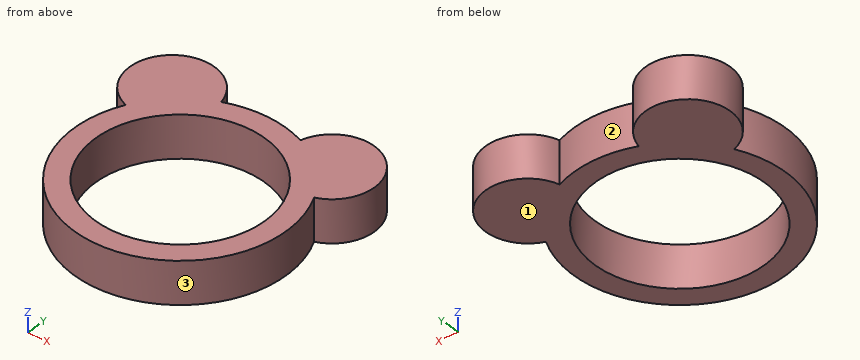
```python
from build123d import *

# Parameters (mm, degrees)
CYLINDER001_R     = 4
CYLINDER001_DEPTH = 5
CYLINDER003_R     = 2
CYLINDER003_DEPTH = 2
CYLINDER002_R     = 2
CYLINDER002_DEPTH = 2
CYLINDER_R        = 5
CYLINDER_DEPTH    = 2


with BuildPart() as interior:
    # Cylinder001 → Cylinder001 (new body)
    with BuildSketch(Plane.XY.offset(-1.53)):
        Circle(CYLINDER001_R)
    extrude(amount=CYLINDER001_DEPTH)


with BuildPart() as obj1:
    # Cylinder003 → Cylinder003 (new body)
    with BuildSketch(Plane(origin=(3.74, 4.15, 0), x_dir=(1, 0, 0), z_dir=(0, 0, 1))):
        Circle(CYLINDER003_R)
    extrude(amount=CYLINDER003_DEPTH)


with BuildPart() as cut001:
    # Cylinder002 → Cylinder002 (new body)
    with BuildSketch(Plane(origin=(-3.86, 4.15, 0), x_dir=(1, 0, 0), z_dir=(0, 0, 1))):
        Circle(CYLINDER002_R)
    extrude(amount=CYLINDER002_DEPTH)

    # Fusion: union obj1
    add(obj1.part)

    # Cut001: cut Interior
    add(interior.part, mode=Mode.SUBTRACT)


with BuildPart() as fusion001:
    # Cylinder → Cylinder (new body)
    with BuildSketch(Plane.XY):
        Circle(CYLINDER_R)
    extrude(amount=CYLINDER_DEPTH)

    # Cut: cut Interior
    add(interior.part, mode=Mode.SUBTRACT)

    # Fusion001: union Cut001
    add(cut001.part)


solid = fusion001.part
```
Can you work these out from the model? Positions are in its coordinate system, mm. Face numbers are marked on the shaded views. Give positions to 0.01 mm unless a question says otherwise; leave off trailing zeros. Order: outer loops, then holes, each group sorted by start corner. A loop starts at its lowest first (then second) coordinate and runs counter-clockwise, first axis right, second up. Notation, with made-up numbers: (85, 25.25) - (136, 25.25) arc R12 ccw to (136, 32.25) - close; hole circle Ø6 at (-3.5, 0). An arc over 180 degrees is marked (long way). Use a Markdown table: item, result. Add a question column.
Q1. If we section it at C-C on z = 0.15: Write out the boundary of the cut face in (x, y).
Q2. I'm going to push flat-ended pins straight in: pin 1 (6.5 mm diameter, centred on x = 0, y = 0, fed in from -Z); pin 2 (1 mm diameter, centred on y = -1.5, z = 0, fed in from -X). Where does each tip first touch, or does it pass through?
Q3. Please list where these lines run through material, in increasing order: line 1 along Y through (x, z) = (0, 1); line 2 along Y through (x, z) = (-1, 0.9); line 3 along X through (y, z) = (3.5, 1.85).
Q4. If we section it at A-A on y = 0: Write out the boundary of the cut face in (x, z), plus the area to 3 significant figures.
Q5. If we mould it in two halves opening along X, with no side actions, what happens to the marked faces 1, 2 and 3? For each: released by +X, released by -X, zero draft, split by the parting line, or undercut.
Answers follow:
| question | item | result |
|---|---|---|
| 1 | outline | (-4.47, 2.24) arc R5 ccw (long way) to (4.45, 2.28) arc R2 ccw (long way) to (1.81, 4.66) arc R5 ccw to (-1.92, 4.62) arc R2 ccw (long way) to start; hole circle Ø8 at (0, 0) |
| 2 | pin 1 | passes through |
| 2 | pin 2 | stops at x = -4.9 |
| 3 | line 1 | y = -5 to -4, 4 to 5 |
| 3 | line 2 | y = -4.9 to -3.87, 3.87 to 4.9 |
| 3 | line 3 | x = -5.75 to -1.94, 1.94 to 5.63 |
| 4 | outline | (-5, 0) - (-4, 0) - (-4, 2) - (-5, 2) - close; (4, 0) - (5, 0) - (5, 2) - (4, 2) - close |
| 4 | area | 4.00 mm^2 |
| 5 | face 1 | zero draft |
| 5 | face 2 | undercut |
| 5 | face 3 | split by the parting line |
